```python
from build123d import *

# Parameters (mm, degrees)
SKETCH1_R           = 4.7625
BOSS_EXTRUDE1_DEPTH = 6.35


with BuildPart() as part:
    # Sketch1 → Boss-Extrude1 (new body)
    with BuildSketch(Plane(origin=(0, 0, 0), x_dir=(0, 0, -1), z_dir=(1, 0, 0))):
        with BuildLine():
            Line((6.35, 0), (273.05, 0))
            ThreePointArc((273.05, 0), (277.540128061, 1.859871939), (279.4, 6.35))
            Line((279.4, 6.35), (279.4, 120.65))
            ThreePointArc((279.4, 120.65), (277.540128061, 125.140128061), (273.05, 127))
            Line((273.05, 127), (55.42230509, 127))
            ThreePointArc((55.42230509, 127), (45.702145908, 125.066540126), (37.461792847, 119.560512242))
            Line((37.461792847, 119.560512242), (7.439487758, 89.538207153))
            ThreePointArc((7.439487758, 89.538207153), (1.933459874, 81.297854092), (0, 71.57769491))
            Line((0, 71.57769491), (0, 6.35))
            ThreePointArc((0, 6.35), (1.859871939, 1.859871939), (6.35, 0))
        make_face()
        with Locations((38.1, 25.4)):
            Circle(SKETCH1_R, mode=Mode.SUBTRACT)
        with Locations((126.134831311, 37.772488675)):
            Circle(SKETCH1_R, mode=Mode.SUBTRACT)
    extrude(amount=BOSS_EXTRUDE1_DEPTH)


solid = part.part
```
Check sheet for the modelled part. Datum: model origin and axes. Units: mm. Give positions to 0.01 mm unless a question says otherwise; leave off trailing zeros. Order: outer loops, then holes, each group sorted by start corner. A loop starts at its lowest first (then second) coordinate and runs counter-clockwise, first axis right, second up. Notation, with made-up numbers: (-30.75, 65) -> (8.25, 65) arc R12 ccw to (8.25, 73) -> close; hole circle Ø10 at (11, -6). An arc over 180 degrees is marked (long way). Use CSV: the item, a comma, the result in double quotes. Start each with the question number.
1) Sectioned sample at B-B, the plane x = 2. Give the number of separate pieces and of enclosed holes in the cut face, plus the area to 3 significant figures.
2) Sectioned sample at A-A, the plane y = 25.4. Record the boundary of the cut face in (x, z).
3) Mould release check, pull along Z, two halves, no side actions. Record for faces 1 (the face through (3.13, 39.2, -130.68)), 2 (the face through (3, 39, 0)), 3 (the face through (3.131, 26.831, -42.643)), 4 (the face through (0, 64, -138)): released by +Z, released by -Z, zero draft, split by the parting line, or undercut.
4) Sectioned sample at C-C, the plane y = 106.5. Record the boundary of the cut face in (x, z), plus the area to 3 significant figures.
5) Material ranges on line 1 (Z direction, x = 3.5, y = 38.5); line 2 (Y direction, x = 2, z = -38.1); line 3 (Z direction, x = 3, y = 34), recorded low to high. Write a range as from..to.
Recorded:
1,separate pieces,"1"
1,enclosed holes,"2"
1,area,"34,300 mm2"
2,outline,"(0, -279.4) -> (6.35, -279.4) -> (6.35, -42.86) -> (0, -42.86) -> close; (0, -33.34) -> (6.35, -33.34) -> (6.35, 0) -> (0, 0) -> close"
3,face 1,"undercut"
3,face 2,"released by +Z"
3,face 3,"undercut"
3,face 4,"zero draft"
4,outline,"(0, -279.4) -> (6.35, -279.4) -> (6.35, -24.4) -> (0, -24.4) -> close"
4,area,"1,620 mm2"
5,line 1,"-279.4..-130.84, -121.43..0"
5,line 2,"0..20.64, 30.16..120.18"
5,line 3,"-279.4..-129.04, -123.23..0"
